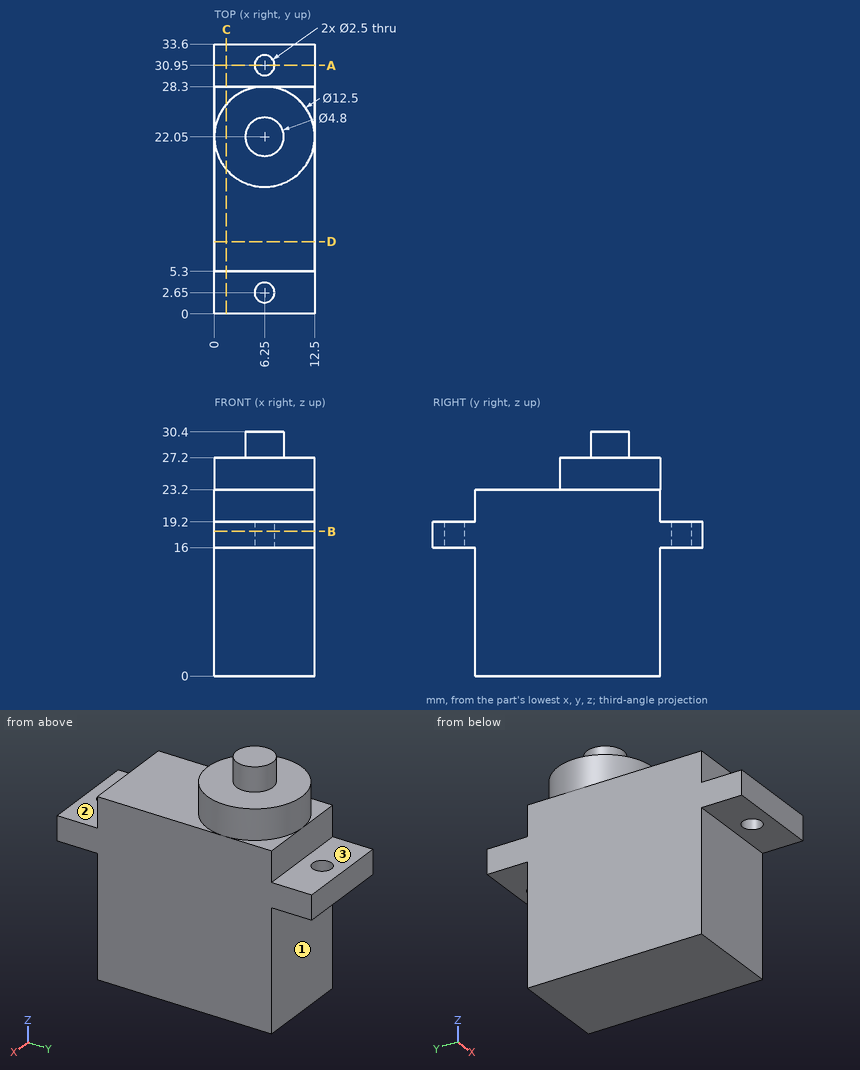
The drawing under review shows one solid part. Ordinate dimensions are in mm from its lowest x, y, z. A direction names the side the tool comes from. Round coordinates to 2 decimals unless told otherwise and drop trailing zeros. Write each loop counter-clockwise with the first axis right and the second up, starting at its lowest first coordinate (ties: lowest second). Pieces come first, ordered by that corner, then holes. Notation, with made-up numbers: (-24.75, 54) -> (-1.75, 54) arc R15 cw to (-1.75, 79) -> close; hole circle Ø9 at (60.25, -5). An arc over 180 degrees is marked (long way). Put each result on its own line as item: value.
Q1. Consider section A-A on y = 30.95. State the section outline as (x, z) points, and give its area (3 significant figures).
Determined:
outline: (0, 16) -> (5, 16) -> (5, 19.2) -> (0, 19.2) -> close; (7.5, 16) -> (12.5, 16) -> (12.5, 19.2) -> (7.5, 19.2) -> close
area: 32.0 mm^2
Q2. Consider section C-C on x = 1.5. State the section outline as (y, z) points.
Determined:
outline: (0, 16) -> (5.3, 16) -> (5.3, 0) -> (28.3, 0) -> (28.3, 16) -> (33.6, 16) -> (33.6, 19.2) -> (28.3, 19.2) -> (28.3, 23.2) -> (26.11, 23.2) -> (26.11, 27.2) -> (17.99, 27.2) -> (17.99, 23.2) -> (5.3, 23.2) -> (5.3, 19.2) -> (0, 19.2) -> close
Q3. To check wall thickness, follow L1, parallel to Y at x = 6.25, z = 17.4; L2, parallel to Y at x = 6.75, z = 19; L3, parallel to X at y = 30.95, z = 18.55. State the ranges of each line that lie inside material, in increasing order. Write a range as [from, to].
Determined:
L1: y = [0, 1.4], [3.9, 29.7], [32.2, 33.6]
L2: y = [0, 1.5], [3.8, 29.8], [32.1, 33.6]
L3: x = [0, 5], [7.5, 12.5]
Q4. Consider section B-B on z = 18. State the section outline as (x, y) points.
Determined:
outline: (0, 0) -> (12.5, 0) -> (12.5, 33.6) -> (0, 33.6) -> close; hole circle Ø2.5 at (6.25, 2.65); hole circle Ø2.5 at (6.25, 30.95)
Q5. Machinability: for the marked faces 1, 2 and 3, which of the approach directions +Z, -Z, +X, -X, +Y, -Y give a long, thin tool a straight path to every point of the face, cutting with its end or side? Answer none if there is none.
Determined:
face 1: -Z, +X, -X, +Y
face 2: +Z, +X, -X, -Y
face 3: +Z, +X, -X, +Y
Q6. Clearance check with flat-ended pins moving along their axes: pin 1 Ø1 at (x, y) = (10.5, 26) entering from -Z; pin 2 Ø4.5 at (x, z) = (6, 21.5) entering from +Y; pin 3 Ø1.2 at (x, z) = (3.5, 20.5) entering from -Y; pin 4 Ø2 at (x, y) = (6.25, 2.65) entering from -Z. State where each tip first meets the part, or that it passes through.
Determined:
pin 1: stops at z = 0
pin 2: stops at y = 28.3
pin 3: stops at y = 5.3
pin 4: passes through
Q7. Consider section D-D on y = 9. State the section outline as (x, z) points.
Determined:
outline: (0, 0) -> (12.5, 0) -> (12.5, 23.2) -> (0, 23.2) -> close
